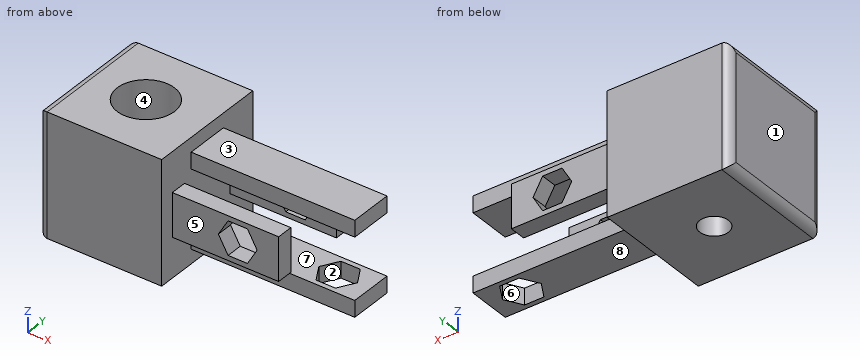
```python
from build123d import *

# Parameters (mm, degrees)
ESBO_O1_W                  = 15
ESBO_O1_H                  = 15
ESBO_O1_R                  = 3.5
RESSALTO_EXTRUS_O1_DEPTH   = 7.5
RESSALTO_EXTRUS_O2_START   = -7.5
ESBO_O1_3_R                = 3.5
ESBO_O1_3_R_2              = 1.75
RESSALTO_EXTRUS_O2_DEPTH   = 3
ESBO_O2_3_R                = 3.5
ESBO_O2_3_R_2              = 1.6
RESSALTO_EXTRUS_O3_DEPTH   = 3
ESBO_O4_3_R                = 3.5
ESBO_O4_3_R_2              = 1.6
RESSALTO_EXTRUS_O4_DEPTH   = 3
ESBO_O6_W                  = 5.3
ESBO_O6_H                  = 2
ESBO_O6_W_2                = 2
ESBO_O6_H_2                = 5.3
RESSALTO_EXTRUS_O5_DEPTH   = 20
ESBO_O7_W                  = 7
ESBO_O7_H                  = 5.3
CORTE_EXTRUS_O3_DEPTH      = 1
CORTE_EXTRUS_O3_DEPTH_BACK = 16
CORTE_EXTRUS_O4_DEPTH      = 3
FILETE1_R                  = 1


with BuildPart() as part:
    # Esboço1 → Ressalto-extrusão1 (new body, symmetric)
    with BuildSketch(Plane.XY):
        Rectangle(ESBO_O1_W, ESBO_O1_H)
        Circle(ESBO_O1_R, mode=Mode.SUBTRACT)
    extrude(amount=RESSALTO_EXTRUS_O1_DEPTH, both=True)

    # Esboço1<3> → Ressalto-extrusão2 (add)
    with BuildSketch(Plane.XY.offset(RESSALTO_EXTRUS_O2_START)):
        Circle(ESBO_O1_3_R)
        Circle(ESBO_O1_3_R_2, mode=Mode.SUBTRACT)
    extrude(amount=RESSALTO_EXTRUS_O2_DEPTH)

    # Esboço2<3> → Ressalto-extrusão3 (add)
    with BuildSketch(Plane(origin=(7.5, 0, 0), x_dir=(0, 0, -1), z_dir=(1, 0, 0))):
        Circle(ESBO_O2_3_R)
        Circle(ESBO_O2_3_R_2, mode=Mode.SUBTRACT)
    extrude(amount=-RESSALTO_EXTRUS_O3_DEPTH)

    # Esboço4<3> → Ressalto-extrusão4 (add)
    with BuildSketch(Plane(origin=(0, 7.5, 0), x_dir=(1, 0, 0), z_dir=(0, 1, 0))):
        Circle(ESBO_O4_3_R)
        Circle(ESBO_O4_3_R_2, mode=Mode.SUBTRACT)
    extrude(amount=-RESSALTO_EXTRUS_O4_DEPTH)

    # Esboço6 → Ressalto-extrusão5 (add)
    with BuildSketch(Plane(origin=(7.5, 0, 0), x_dir=(0, 0, -1), z_dir=(1, 0, 0))):
        with Locations((0, 4.75)):
            Rectangle(ESBO_O6_W, ESBO_O6_H)
        with Locations((4.75, 0)):
            Rectangle(ESBO_O6_W_2, ESBO_O6_H_2)
        with Locations((0, -4.75)):
            Rectangle(ESBO_O6_W, ESBO_O6_H)
        with Locations((-4.75, 0)):
            Rectangle(ESBO_O6_W_2, ESBO_O6_H_2)
    extrude(amount=RESSALTO_EXTRUS_O5_DEPTH)

    # Esboço7 → Corte-extrusão3 (cut, two sides)
    with BuildSketch(Plane.XZ.offset(7.5)) as corte_extrus_o3_sk:
        with Locations((24, 0)):
            Rectangle(ESBO_O7_W, ESBO_O7_H)
        Polygon((17.867136104, 0), (16.683568052, 2.05), (14.316431948, 2.05), (13.132863896, 0), (14.316431948, -2.05), (16.683568052, -2.05), align=None)
    extrude(amount=CORTE_EXTRUS_O3_DEPTH, mode=Mode.SUBTRACT)
    extrude(corte_extrus_o3_sk.sketch, amount=-CORTE_EXTRUS_O3_DEPTH_BACK, mode=Mode.SUBTRACT)

    # Esboço8 → Corte-extrusão4 (cut)
    with BuildSketch(Plane(origin=(0, 0, -5.75), x_dir=(-1, 0, 0), z_dir=(0, 0, -1))):
        Polygon((-25.867136104, 0), (-24.683568052, -2.05), (-22.316431948, -2.05), (-21.132863896, 0), (-22.316431948, 2.05), (-24.683568052, 2.05), align=None)
    extrude(amount=-CORTE_EXTRUS_O4_DEPTH, mode=Mode.SUBTRACT)

    # Filete1
    filete1_edges = [part.edges().sort_by_distance(p)[0] for p in [
        (-7.5, -7.5, 0),
        (-7.5, 7.5, 0),
        (-7.5, 0, 7.5),
        (-7.5, 0, -7.5),
    ]]
    fillet(filete1_edges, radius=FILETE1_R)


solid = part.part
```
Model file for the job. Use its own axes, mm. Face numbers are marked on the shaded views. A direction names the side the tool comes from. Coordinates: 2 decimals unless noted, no trailing zeros. Order: outer loops, then holes, each group sorted by start corner. A loop starts at its lowest first (then second) coordinate and runs counter-clockwise, first axis right, second up. Notation, with made-up numbers: (-36, 45.25) - (-31, 45.25) arc R17 cw to (-31, 51.25) - close; hole circle Ø10 at (80, 58.25). An arc over 180 degrees is marked (long way). Return JSON: item names as keys, results as strings. Group by question number.
1) Saw through at B-B, the plane x = 0. Write the cut outline in (y, z), plus the area to 4 significant figures.
2) Mould opens along X. For the marked faces 1, 2, 3 and 4 say: released by +X, released by -X, zero draft, split by the parting line, or undercut.
3) Tool access for the marked faces 5, 6, 7 and 8: list every direction of +Z, -Z, +X, -X, +Y, -Y with a clear straight run to the whole face (end or side of a thin tool).
4) Probe line 1 (Y direction, x = 0, z = -6.15); line 2 (Y direction, x = 0, z = -1.75); line 3 (Z direction, x = 14.5, y = -0.5). List the from-to ranges inside material, lowest first. Write a range as from..to.
5) Flat gauge pins, fed straight in: P1, Ø1.6, axis at x = 13, y = -5, coming from the +Z side; P2, Ø6, axis at x = 15, z = 0, coming from the +Y side; P3, Ø1.6, axis at x = 11, y = -4.5, coming from the -Z side. Where does each tip first touch, or does it go through?
6) Saw through at A-A, the plane x = 24. Write the cut outline in (y, z).
Values found:
{
 "1": {"outline": "(-7.5, -7.5) - (-1.75, -7.5) - (-1.75, -4.5) - (-3.5, -4.5) - (-3.5, 7.5) - (-7.5, 7.5) - close; (1.75, -7.5) - (7.5, -7.5) - (7.5, 7.5) - (3.5, 7.5) - (3.5, -4.5) - (1.75, -4.5) - close", "area": "130.5 mm²"},
 "2": {"face 1": "released by -X", "face 2": "undercut", "face 3": "zero draft", "face 4": "undercut"},
 "3": {"face 5": "+Z, -Z, +X, -Y", "face 6": "-Z", "face 7": "+X, +Y, -Y", "face 8": "-Z, +X, +Y, -Y"},
 "4": {"line 1": "y = -7.5..-1.75, 1.75..7.5", "line 2": "y = -7.5..-3.5, 3.5..7.5", "line 3": "z = -5.75..-3.75, 3.75..5.75"},
 "5": {"P1": "stops at z = 2.65", "P2": "stops at y = 5.75", "P3": "stops at z = -2.65"},
 "6": {"outline": "(-2.65, -5.75) - (-2.05, -5.75) - (-2.05, -3.75) - (-2.65, -3.75) - close; (-2.65, 3.75) - (2.65, 3.75) - (2.65, 5.75) - (-2.65, 5.75) - close; (2.05, -5.75) - (2.65, -5.75) - (2.65, -3.75) - (2.05, -3.75) - close"}
}
